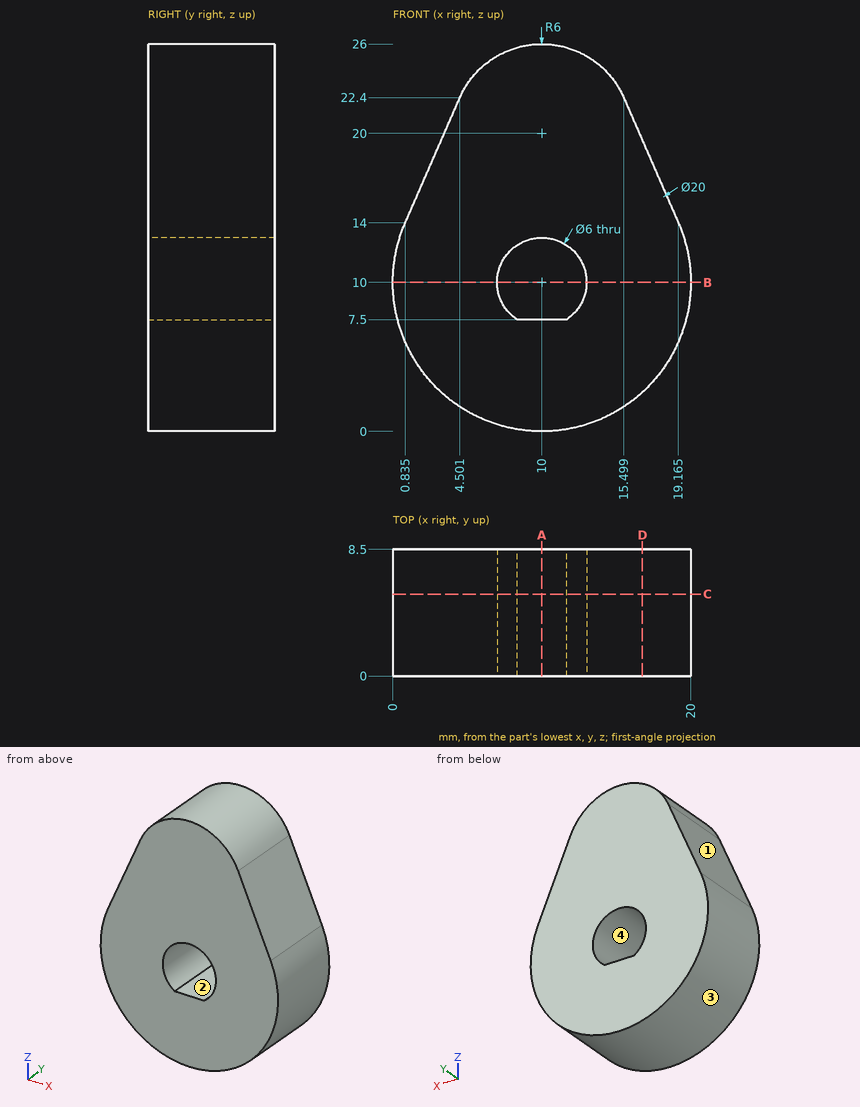
Study the drawing (mm; zero at the part's minimum x, y, z) and answer. Give positions to 0.01 mm unless a question says otherwise; leave off trailing zeros. Order: outer loops, then holes, each group sorted by start corner. A loop starts at its lowest first (then second) coordinate and runs counter-clockwise, first axis right, second up. Notation, with made-up numbers: (31.5, 63.25) - (66.5, 63.25) arc R26 ccw to (66.5, 91.25) - close; hole circle Ø1 at (29.5, -29.75). An arc over 180 degrees is marked (long way). Answer in a Markdown table with one row per item. Add a question column.
Q1. The part is cut by section A-A (x = 10). Determine the outline of the cut face in (y, z), then the cut area to 3 significant figures.
Q2. For a pull along Z with two mould halves and no side action, classify the marked faces 1, 2, 3 and 4 as released by +Z, released by -Z, zero draft, split by the parting line, or undercut.
Q3. The part is cut by section D-D (x = 16.75). Determine the outline of the cut face in (y, z), then the cut area to 3 significant figures.
Q4. The part is cut by section B-B (z = 10). Determine the outline of the cut face in (x, y).
Q5. The part is cut by section C-C (y = 5.5). Determine the outline of the cut face in (x, z) (1 decimal), then the cut area to 3 significant figures.
Q6. Given P1, Ø4, axis at x = 6.5, y = 5, coming from the +Z side, flat-ended and moving along its own axis, determine where the tip first touches the part or whether it passes through.
Q7. Find the intervals of material crossed by line 1 along X through (y, z) = (6, 10); line 2 along Z through (x, y) = (10.5, 0.5); line 3 along X through (y, z) = (1.75, 7.75) (1 decimal), in increasing order. Write a range as [from, to].
Determined:
| question | item | result |
|---|---|---|
| 1 | outline | (0, 0) - (8.5, 0) - (8.5, 7.5) - (0, 7.5) - close; (0, 13) - (8.5, 13) - (8.5, 26) - (0, 26) - close |
| 1 | area | 174 mm² |
| 2 | face 1 | released by +Z |
| 2 | face 2 | undercut |
| 2 | face 3 | split by the parting line |
| 2 | face 4 | undercut |
| 3 | outline | (0, 2.62) - (8.5, 2.62) - (8.5, 19.53) - (0, 19.53) - close |
| 3 | area | 144 mm² |
| 4 | outline | (0, 0) - (7, 0) - (7, 8.5) - (0, 8.5) - close; (13, 0) - (20, 0) - (20, 8.5) - (13, 8.5) - close |
| 5 | outline | (0.8, 14) arc R10 ccw (long way) to (19.2, 14) - (15.5, 22.4) arc R6 ccw to (4.5, 22.4) - close; hole (8.3, 7.5) - (11.7, 7.5) arc R3 ccw (long way) to start |
| 5 | area | 359 mm² |
| 6 | P1 | stops at z = 25.81 |
| 7 | line 1 | x = [0, 7], [13, 20] |
| 7 | line 2 | z = [0.01, 7.5], [12.96, 25.98] |
| 7 | line 3 | x = [0.3, 8], [12, 19.7] |
